Build history of the part. All positions in model axes, mm. A direction names the side the tool comes from. Give positions to 0.01 mm unless a question says otherwise; leave off trailing zeros. Order: outer loops, then holes, each group sorted by start corner. A loop starts at its lowest first (then second) coordinate and runs counter-clockwise, first axis right, second up. Notation, with made-up numbers: (20, 50) - (69, 50) arc R29 cw to (69, 85) - close; hole circle Ø1 at (45, 85.25). An arc over 180 degrees is marked (long way). Use a Markdown table: item, result. Add a question column.
(1) Slice it at C-C (z = -32). Write the cut outline in (x, y), then the cut area to 3 significant figures.
(2) Which spindle directions (+Z, -Z, +X, -X, +Y, -Y) get a long thin tool onto all of the face, cutting with end or side? Do faces 1 (the face through (35.34, 29.993, -33.084)), 2 (the face through (36, 18, 9)), 3 (the face through (28.5, 32.3, 0)). Say none if no direction does.
(3) Slice it at B-B (y = 10.5). Count the separate pieces of the cut face and the enclosed holes in it, then the cut area to 3 significant figures.
(4) Slice it at A-A (z = -12). Write the cut outline in (x, y), then the cut area to 3 significant figures.
(5) Flat gauge pins, fed straight in: pin 1 (6 mm diameter, centred on y = 9.5, z = 12, fed in from -X); pin 2 (1 mm diameter, centred on y = 24, z = -27.5, fed in from +X); pin 3 (4 mm diameter, centred on x = 35.5, y = 10, fed in from -Z). Where does each tip first touch, or does it go through?
(6) Mould opens along X. For faces 4 (the face through (36.66, 29.993, 8.916)), 5 (the face through (0, 16, -12)), 6 (the face through (38.23, 16.27, -12.29)) say: +X half, -X half, draft (parallel to the pull), parting line (faces both ways), or undercut.
(7) Wall check: line 1 (X direction, y = 17.5, z = -12); line 2 (X direction, y = 14.5, z = -11); line 3 (X direction, y = 11.5, z = -15). Give the ranges that are in metal, low to high.
from build123d import *

# Parameters (mm, degrees)
SKETCH_2_W      = 72
SKETCH_2_H      = 24
SKETCH_2_R      = 6.05
SKETCH_2_R_2    = 2.25
EXTRUDE_1_DEPTH = 33
FILLET_1_R      = 3
EXTRUDE_2_DEPTH = 18
EXTRUDE_START   = 18
EXTRUDE_3_DEPTH = 18
FILLET_2_R      = 3


with BuildPart() as part:
    # 草圖2 → 填料-伸長1 (new body)
    with BuildSketch(Plane(origin=(0, 0, 0), x_dir=(1, 0, 0), z_dir=(0, 1, 0))):
        with Locations((36, 12)):
            Rectangle(SKETCH_2_W, SKETCH_2_H)
        with Locations(Location((9, 12, 0), (0, 0, 270))):
            Circle(SKETCH_2_R, mode=Mode.SUBTRACT)
        with Locations(Location((63, 12, 0), (0, 0, 270))):
            Circle(SKETCH_2_R, mode=Mode.SUBTRACT)
        with Locations(Location((36, 12, 0), (0, 0, 270))):
            Circle(SKETCH_2_R_2, mode=Mode.SUBTRACT)
    extrude(amount=EXTRUDE_1_DEPTH)

    # 圓角1
    fillet_1_edges = [part.edges().sort_by_distance(p)[0] for p in [
        (0, 16.5, -24),
        (72, 16.5, -24),
        (72, 16.5, 0),
        (0, 16.5, 0),
    ]]
    fillet(fillet_1_edges, radius=FILLET_1_R)

    # 草圖4 → 填料-伸長2 (add)
    with BuildSketch(Plane.XY):
        with BuildLine():
            ThreePointArc((66, 0), (36, 30), (6, 0))
            Line((6, 0), (18, 0))
            ThreePointArc((18, 0), (36, 18), (54, 0))
            Line((54, 0), (66, 0))
        make_face()
    extrude(amount=EXTRUDE_2_DEPTH)

    # 草圖5 → 填料-伸長3 (add)
    with BuildSketch(Plane(origin=(0, 0, -24), x_dir=(-1, 0, 0), z_dir=(0, 0, -1)).offset(EXTRUDE_START)):
        with BuildLine():
            ThreePointArc((-6, 0), (-36, 30), (-66, 0))
            Line((-66, 0), (-54, 0))
            ThreePointArc((-54, 0), (-36, 18), (-18, 0))
            Line((-18, 0), (-6, 0))
        make_face()
    extrude(amount=-EXTRUDE_3_DEPTH)

    # 圓角2
    fillet_2_edges = [part.edges().sort_by_distance(p)[0] for p in [
        (36, 30, -42),
        (36, 30, -24),
        (36, 30, 18),
        (36, 30, 0),
    ]]
    fillet(fillet_2_edges, radius=FILLET_2_R - 0.0001)  # a hair under: the kernel refuses the full size


solid = part.part
Solution:
| question | item | result |
|---|---|---|
| 1 | outline | (6, 0) - (18, 0) arc R18 cw to (54, 0) - (66, 0) arc R30 ccw to start |
| 1 | area | 905 mm2 |
| 2 | face 1 | -Z, +Y |
| 2 | face 2 | +Z, -Y |
| 2 | face 3 | +Z, +Y |
| 3 | separate pieces | 1 |
| 3 | enclosed holes | 3 |
| 3 | area | 2,450 mm2 |
| 4 | outline | (0, 0) - (2.95, 0) - (2.95, 33) - (0, 33) - close; (15.05, 0) - (33.75, 0) - (33.75, 33) - (15.05, 33) - close; (38.25, 0) - (56.95, 0) - (56.95, 33) - (38.25, 33) - close; (69.05, 0) - (72, 0) - (72, 33) - (69.05, 33) - close |
| 4 | area | 1,430 mm2 |
| 5 | pin 1 | x = 6.71 |
| 5 | pin 2 | x = 54.65 |
| 5 | pin 3 | z = -24 |
| 6 | face 4 | parting line |
| 6 | face 5 | -X half |
| 6 | face 6 | undercut |
| 7 | line 1 | 0 to 2.95, 15.05 to 33.75, 38.25 to 56.95, 69.05 to 72 |
| 7 | line 2 | 0 to 3.03, 14.97 to 33.98, 38.02 to 57.03, 68.97 to 72 |
| 7 | line 3 | 0 to 3.75, 14.25 to 57.75, 68.25 to 72 |
